```python
from build123d import *

# Parameters (mm, degrees)
F0_W      = 31.7
F0_H      = 31.7
F1_DEPTH  = 7.9
F3_DEPTH  = 7.901
F4_W      = 7.925
F4_H      = 7.75
F2_W      = 7.925
F2_H      = 7.75
F5_DEPTH  = 8.23
F6_DEPTH  = 8.23
F7_W      = 7.925
F7_H      = 7.75
F8_DEPTH  = 8.23
F10_DEPTH = 7.925
F12_DEPTH = 7.925


with BuildPart() as f1:
    # F0 (on Top) → F1 (new body)
    with BuildSketch(Plane.XY):
        with Locations((15.85, 15.85)):
            Rectangle(F0_W, F0_H)
    extrude(amount=F1_DEPTH)

    # F2 (on face) → F3 (cut, through all)
    with BuildSketch(Plane.XY.offset(7.9)):
        Polygon((15.85, 0), (31.7, 0), (31.7, 23.95), (23.775, 23.95), (15.85, 23.95), align=None)
    extrude(amount=-F3_DEPTH, mode=Mode.SUBTRACT)

    # F4 (on face) + F2 (on face) → F5 (join)
    with BuildSketch(Plane.XY.offset(7.9)):
        with Locations((27.7375, 27.825)):
            Rectangle(F4_W, F4_H)
    with BuildSketch(Plane.XY.offset(7.9)):
        with Locations((27.7375, 27.825)):
            Rectangle(F2_W, F2_H)
    extrude(amount=F5_DEPTH)

    # F2 (on face) → F6 (join)
    with BuildSketch(Plane.XY.offset(7.9)):
        Polygon((0, 0), (15.85, 0), (15.85, 23.95), (23.775, 23.95), (23.775, 31.7), (0, 31.7), align=None)
    extrude(amount=F6_DEPTH)

    # F7 (on face) → F8 (cut)
    with BuildSketch(Plane.XY.offset(16.13)):
        with Locations((19.8125, 27.825)):
            Rectangle(F7_W, F7_H)
        Polygon((0, 0), (7.925, 0), (7.925, 7.925), (15.85, 7.925), (15.85, 15.85), (0, 15.85), align=None)
    extrude(amount=-F8_DEPTH, mode=Mode.SUBTRACT)

    # F9 (on face) → F10 (join, through all)
    with BuildSketch(Plane.YZ.offset(15.85)):
        Polygon((15.85, 7.9), (7.925, 16.13), (7.925, 7.9), align=None)
    extrude(amount=-F10_DEPTH)

    # F11 (on face) → F12 (cut, through all)
    with BuildSketch(Plane.YZ.offset(15.85)):
        Polygon((23.95, 0), (31.7, 7.9), (23.95, 7.9), align=None)
    extrude(amount=F12_DEPTH, mode=Mode.SUBTRACT)


solid = f1.part
```
The model under review builds one solid part; all positions refer to its coordinate system, in mm. A direction names the side the tool comes from. Round coordinates to 2 decimals unless told otherwise and drop trailing zeros. Order: outer loops, then holes, each group sorted by start corner. A loop starts at its lowest first (then second) coordinate and runs counter-clockwise, first axis right, second up.
Item 1: Add section D-D, the plane y = 3.5. State the section outline as (x, z) points (3 decimals), and give its area (3 significant figures).
Working result:
outline: (0, 0) - (15.85, 0) - (15.85, 16.13) - (7.925, 16.13) - (7.925, 7.9) - (0, 7.9) - close
area: 190 mm2
Item 2: Machinability: for faces 1 (the flat face through (4, 8, 7.9)), 2 (the flat face through (8, 15.85, 12)), 3 (the flat face through (28, 23.95, 8)), 4 (the flat face through (23.775, 28, 10)), which of the approach directions +Z, -Z, +X, -X, +Y, -Y give a long, thin tool a straight path to every point of the face, cutting with its end or side? Answer none if there is none.
Working result:
face 1: +Z, -X, -Y
face 2: +Z, +X, -X
face 3: +Z, -Z, +X, -Y
face 4: +Z, -Y
Item 3: Draft analysis for pull direction X (two halves, no side actions). For faces 5 (the flat face through (31.7, 28, 8)), 6 (the flat face through (8, 24, 16.13)), 7 (the flat face through (19.757, 27.771, 3.895)), state which applies: released by +X, released by -X, zero draft, split by the parting line, or undercut.
Working result:
face 5: released by +X
face 6: zero draft
face 7: undercut
Item 4: For pin 1 (8.5 mm diameter, centred on x = 28.5, z = 11, fed in from -Y); pin 2 (4 mm diameter, centred on x = 5.5, y = 7.5, fed in from +Z); pin 3 (1 mm diameter, centred on y = 21, z = 7, fed in from +X), all flat-tipped, find the tip position at first contact; note any pin that passes through.
Working result:
pin 1: stops at y = 23.95
pin 2: stops at z = 7.9
pin 3: stops at x = 15.85
Item 5: To check wall thickness, follow probe 1 along X at (y, z) = (30, 11.5) (3 decimals); probe 2 along X at (y, z) = (23.5, 2.5); probe 3 along Y at (x, z) = (27, 1.75). State the ranges of each line that lie inside material, in increasing order.
Working result:
probe 1: x = 0 to 15.85, 23.775 to 31.7
probe 2: x = 0 to 15.85
probe 3: y = 23.95 to 31.7
Item 6: Add section B-B, the plane z = 13.25. State the section outline as (x, y) points (3 decimals), and give its area (3 significant figures).
Working result:
outline: (0, 15.85) - (15.85, 15.85) - (15.85, 31.7) - (0, 31.7) - close; (7.925, 0) - (15.85, 0) - (15.85, 10.698) - (7.925, 10.698) - close; (23.775, 23.95) - (31.7, 23.95) - (31.7, 31.7) - (23.775, 31.7) - close
area: 397 mm2
Item 7: Add section A-A, the plane x = 13.5. State the section outline as (y, z) points (3 decimals), and give its area (3 significant figures).
Working result:
outline: (0, 0) - (31.7, 0) - (31.7, 16.13) - (15.85, 16.13) - (15.85, 7.9) - (7.925, 16.13) - (0, 16.13) - close
area: 479 mm2
Item 8: Add section C-C, the plane z = 4.5. State the section outline as (x, y) points (3 decimals), and give its area (3 significant figures).
Working result:
outline: (0, 0) - (15.85, 0) - (15.85, 28.365) - (23.775, 28.365) - (23.775, 23.95) - (31.7, 23.95) - (31.7, 31.7) - (0, 31.7) - close
area: 590 mm2
